Model file for the job. Use its own axes, mm. A direction names the side the tool comes from. Coordinates: 2 decimals unless noted, no trailing zeros. Write each loop counter-clockwise with the first axis right and the second up, starting at its lowest first coordinate (ties: lowest second). Pieces come first, ordered by that corner, then holes. Notation, with made-up numbers: M 37,84.5 L 81,84.5 A25 cw 81,98.5 Z; hole C 63.25,39 d5. An arc over 180 degrees is marked long. Answer in a Markdown table with one row per item. Add a question column.
```python
from build123d import *

# Parameters (mm, degrees)
ESBO_O2_W                = 173
ESBO_O2_H                = 45.2
RESSALTO_EXTRUS_O2_DEPTH = 65.2
ESBO_O3_R                = 57.970457698
RESSALTO_EXTRUS_O3_DEPTH = 20
RESSALTO_EXTRUS_O4_START = -45.2
RESSALTO_EXTRUS_O4_DEPTH = 45.2


# Read off the part's stored shape, not the designer's step: Ressalto-extrusão4
with BuildPart() as part:
    # Esboço2 → Ressalto-extrusão2 (new, symmetric)
    with BuildSketch(Plane(origin=(0, 0, 0), x_dir=(1, 0, 0), z_dir=(0, 1, 0))):
        Rectangle(ESBO_O2_W, ESBO_O2_H)
    extrude(amount=RESSALTO_EXTRUS_O2_DEPTH, both=True)

    # Esboço3 → Ressalto-extrusão3 (add)
    with BuildSketch(Plane.XY.offset(22.6)):
        with Locations((-17.919078136, -1.804884681)):
            Circle(ESBO_O3_R)
    extrude(amount=RESSALTO_EXTRUS_O3_DEPTH)

    # Ressalto-extrusão4 outline → Ressalto-extrusão4 (add)
    with BuildSketch(Plane.XY.offset(22.6).offset(RESSALTO_EXTRUS_O4_START)):
        with BuildLine():
            Line((102.68744208, 77.672367144), (93.883087158, 68.853831482))
            Line((93.883087158, 68.853831482), (92.930908203, 67.948153687))
            Line((92.930908203, 67.948153687), (92.052246094, 67.253565979))
            Line((92.052246094, 67.253565979), (91.246276855, 66.845568848))
            Line((91.246276855, 66.845568848), (90.411560059, 66.271777344))
            Line((90.411560059, 66.271777344), (87.657562256, 65.351000977))
            Line((87.657562256, 65.351000977), (86.5, 65.2))
            Line((86.5, 65.2), (86.5, -65.2))
            Line((86.5, -65.2), (93.839447021, -65.336684036))
            Line((93.839447021, -65.336684036), (95.128540039, -65.774876404))
            Line((95.128540039, -65.774876404), (95.626312256, -65.865172195))
            Line((95.626312256, -65.865172195), (97.838317871, -67.1335495))
            Line((97.838317871, -67.1335495), (103.111968994, -71.512766647))
            Line((103.111968994, -71.512766647), (104.284179687, -71.844658661))
            Line((104.284179687, -71.844658661), (105.016326904, -72.192253876))
            Line((105.016326904, -72.192253876), (106.758210561, -72.501532079))
            Line((106.758210561, -72.501532079), (127.042376704, -72.501532079))
            Line((127.042376704, -72.501532079), (128.748016357, -72.237250137))
            Line((128.748016357, -72.237250137), (129.333953857, -71.920157242))
            Line((129.333953857, -71.920157242), (130.505584717, -71.542965698))
            Line((130.505584717, -71.542965698), (132.116973877, -70.621580887))
            Line((132.116973877, -70.621580887), (132.908325195, -70.379986572))
            Line((132.908325195, -70.379986572), (133.581878662, -70.455786514))
            ThreePointArc((133.581878662, -70.455786514), (136.426489502, -71.540170383), (139.104858398, -70.09309082))
            Line((139.104858398, -70.09309082), (144.451446533, -57.847529221))
            ThreePointArc((144.451446533, -57.847529221), (143.532086949, -55.594745414), (141.463348389, -54.313895035))
            Line((141.463348389, -54.313895035), (141.155700684, -53.921302605))
            Line((141.155700684, -53.921302605), (141.155700684, -52.985422897))
            Line((141.155700684, -52.985422897), (141.8878479, -50.116176057))
            Line((141.8878479, -50.116176057), (142.04901123, -47.851521599))
            Line((142.04901123, -47.851521599), (142.561706543, -42.41532402))
            Line((142.561706543, -42.41532402), (142.217758179, -36.926730919))
            Line((142.217758179, -36.926730919), (141.770965576, -33.015906143))
            Line((141.770965576, -33.015906143), (131.194091797, 22.060099792))
            Line((131.194091797, 22.060099792), (130.901397705, 24.174060059))
            Line((130.901397705, 24.174060059), (130.286132812, 26.96738739))
            Line((130.286132812, 26.96738739), (130.286132812, 31.270747375))
            Line((130.286132812, 31.270747375), (131.20904541, 35.347880554))
            Line((131.20904541, 35.347880554), (133.098449707, 39.741893005))
            Line((133.098449707, 39.741893005), (133.699371338, 41.055262756))
            Line((133.699371338, 41.055262756), (133.97769165, 41.886050415))
            Line((133.97769165, 41.886050415), (134.49041748, 42.821932983))
            Line((134.49041748, 42.821932983), (135.134979248, 44.815394592))
            Line((135.134979248, 44.815394592), (135.427642822, 45.69118042))
            Line((135.427642822, 45.69118042), (135.632751465, 46.974353027))
            Line((135.632751465, 46.974353027), (135.60345459, 53.694026184))
            Line((135.60345459, 53.694026184), (135.515838623, 59.205119324))
            Line((135.515838623, 59.205119324), (135.354400635, 60.790583801))
            Line((135.354400635, 60.790583801), (134.665893555, 63.161540222))
            Line((134.665893555, 63.161540222), (134.54901123, 63.659831238))
            Line((134.54901123, 63.659831238), (134.065307617, 64.490313721))
            Line((134.065307617, 64.490313721), (133.684417725, 65.441600037))
            Line((133.684417725, 65.441600037), (132.36630249, 67.208262634))
            Line((132.36630249, 67.208262634), (131.38482666, 68.355540466))
            Line((131.38482666, 68.355540466), (123.254638672, 76.434184265))
            Line((123.254638672, 76.434184265), (122.302154541, 77.249568176))
            Line((122.302154541, 77.249568176), (120.544555664, 78.200854492))
            Line((120.544555664, 78.200854492), (120.134399414, 78.668643188))
            ThreePointArc((120.134399414, 78.668643188), (119.353688391, 81.369611441), (116.808776855, 82.5646698))
            Line((116.808776855, 82.5646698), (106.483274703, 82.583373499))
            ThreePointArc((106.483274703, 82.583373499), (103.379795658, 81.059678188), (102.68744208, 77.672367144))
        make_face()
        with BuildLine():
            Line((-128.748016357, -72.237250137), (-127.042376704, -72.501532079))
            Line((-127.042376704, -72.501532079), (-106.758210561, -72.501532079))
            Line((-106.758210561, -72.501532079), (-105.016326904, -72.192253876))
            Line((-105.016326904, -72.192253876), (-104.284179688, -71.844658661))
            Line((-104.284179688, -71.844658661), (-103.111968994, -71.512766647))
            Line((-103.111968994, -71.512766647), (-97.838317871, -67.1335495))
            Line((-97.838317871, -67.1335495), (-95.626312256, -65.865172195))
            Line((-95.626312256, -65.865172195), (-95.128540039, -65.774876404))
            Line((-95.128540039, -65.774876404), (-93.839447021, -65.336684036))
            Line((-93.839447021, -65.336684036), (-86.5, -65.2))
            Line((-86.5, -65.2), (-86.5, 65.2))
            Line((-86.5, 65.2), (-87.657562256, 65.351000977))
            Line((-87.657562256, 65.351000977), (-90.411560059, 66.271777344))
            Line((-90.411560059, 66.271777344), (-91.246276855, 66.845568848))
            Line((-91.246276855, 66.845568848), (-92.052246094, 67.253565979))
            Line((-92.052246094, 67.253565979), (-92.930908203, 67.948153687))
            Line((-92.930908203, 67.948153687), (-93.883087158, 68.853831482))
            Line((-93.883087158, 68.853831482), (-102.68744208, 77.672367144))
            ThreePointArc((-102.68744208, 77.672367144), (-103.379795658, 81.059678188), (-106.483274703, 82.583373499))
            Line((-106.483274703, 82.583373499), (-116.808776855, 82.5646698))
            ThreePointArc((-116.808776855, 82.5646698), (-119.353688391, 81.369611441), (-120.134399414, 78.668643188))
            Line((-120.134399414, 78.668643188), (-120.544555664, 78.200854492))
            Line((-120.544555664, 78.200854492), (-122.302154541, 77.249568176))
            Line((-122.302154541, 77.249568176), (-123.254638672, 76.434184265))
            Line((-123.254638672, 76.434184265), (-131.38482666, 68.355540466))
            Line((-131.38482666, 68.355540466), (-132.36630249, 67.208262634))
            Line((-132.36630249, 67.208262634), (-133.684417725, 65.441600037))
            Line((-133.684417725, 65.441600037), (-134.065307617, 64.490313721))
            Line((-134.065307617, 64.490313721), (-134.54901123, 63.659831238))
            Line((-134.54901123, 63.659831238), (-134.665893555, 63.161540222))
            Line((-134.665893555, 63.161540222), (-135.354400635, 60.790583801))
            Line((-135.354400635, 60.790583801), (-135.515838623, 59.205119324))
            Line((-135.515838623, 59.205119324), (-135.60345459, 53.694026184))
            Line((-135.60345459, 53.694026184), (-135.632751465, 46.974353027))
            Line((-135.632751465, 46.974353027), (-135.427642822, 45.69118042))
            Line((-135.427642822, 45.69118042), (-135.134979248, 44.815394592))
            Line((-135.134979248, 44.815394592), (-134.49041748, 42.821932983))
            Line((-134.49041748, 42.821932983), (-133.97769165, 41.886050415))
            Line((-133.97769165, 41.886050415), (-133.699371338, 41.055262756))
            Line((-133.699371338, 41.055262756), (-133.098449707, 39.741893005))
            Line((-133.098449707, 39.741893005), (-131.20904541, 35.347880554))
            Line((-131.20904541, 35.347880554), (-130.286132813, 31.270747375))
            Line((-130.286132813, 31.270747375), (-130.286132812, 26.96738739))
            Line((-130.286132812, 26.96738739), (-130.901397705, 24.174060059))
            Line((-130.901397705, 24.174060059), (-131.194091797, 22.060099792))
            Line((-131.194091797, 22.060099792), (-141.770965576, -33.015906143))
            Line((-141.770965576, -33.015906143), (-142.217758179, -36.926730919))
            Line((-142.217758179, -36.926730919), (-142.561706543, -42.41532402))
            Line((-142.561706543, -42.41532402), (-142.04901123, -47.851521599))
            Line((-142.04901123, -47.851521599), (-141.8878479, -50.116176057))
            Line((-141.8878479, -50.116176057), (-141.155700684, -52.985422897))
            Line((-141.155700684, -52.985422897), (-141.155700684, -53.921302605))
            Line((-141.155700684, -53.921302605), (-141.463348389, -54.313895035))
            ThreePointArc((-141.463348389, -54.313895035), (-143.532086949, -55.594745414), (-144.451446533, -57.847529221))
            Line((-144.451446533, -57.847529221), (-139.104858398, -70.09309082))
            ThreePointArc((-139.104858398, -70.09309082), (-136.426489502, -71.540170383), (-133.581878662, -70.455786514))
            Line((-133.581878662, -70.455786514), (-132.908325195, -70.379986572))
            Line((-132.908325195, -70.379986572), (-132.116973877, -70.621580887))
            Line((-132.116973877, -70.621580887), (-130.505584717, -71.542965698))
            Line((-130.505584717, -71.542965698), (-129.333953857, -71.920157242))
            Line((-129.333953857, -71.920157242), (-128.748016357, -72.237250137))
        make_face()
    extrude(amount=RESSALTO_EXTRUS_O4_DEPTH)


solid = part.part
```
1) Slice it at B-B (x = 36). Give the cut face in (y, z).
2) Slice it at C-C (z = 34.5). Give the cut face in (x, y), then the cut area to 3 significant figures.
3) Drill centre lines: probe 1 along Y at (x, z) = (-29, 8.5); probe 2 along Z at (x, y) = (100.5, 24.5); probe 3 along X at (y, z) = (-66, 20.5). Where is each one in solid material? Low to high.
4) Two-plate mould, pull along Y, no slides. Class faces 1 (the face through (-142.31, -45.1, -0.32)), 2 (the face through (136.383, -71.543, -0.316)), 3 (the face through (-2, 6, -22.6)): released by +Y, released by -Y, zero draft, split by the parting line, or undercut.
5) Which spindle directions (+Z, -Z, +X, -X, +Y, -Y) get a long thin tool onto all of the face, cutting with end or side? Do faces 4 (the face through (100.438, -69.293, -0.316)), 5 (the face through (-136.41, -5.09, -0.32)), 6 (the face through (-142.387, -39.633, -0.316)). Say none if no direction does.
6) Slice it at D-D (x = 112). Give the cut face in (y, z), then the cut area to 3 significant figures.
7) Slice it at A-A (y = -4.5). Give the cut face in (x, z).
8) Flat gauge pins, fed straight in: pin 1 Ø4 at (x, z) = (16.5, 25) entering from -Y; pin 2 Ø3.5 at (y, z) = (28.5, -1) entering from -X; pin 3 Ø12 at (y, z) = (-32.5, 8) entering from -X. Where does each tip first touch, or does it go through?
Ans:
| question | item | result |
|---|---|---|
| 1 | outline | M -65.2,-22.6 L 65.2,-22.6 L 65.2,22.6 L 19.49,22.6 L 19.49,42.6 L -23.1,42.6 L -23.1,22.6 L -65.2,22.6 Z |
| 2 | outline | C -17.92,-1.8 d115.94 |
| 2 | area | 10,600 mm2 |
| 3 | probe 1 | y = -65.2 to 65.2 |
| 3 | probe 2 | z = -22.6 to 22.6 |
| 3 | probe 3 | x = -140.89 to -95.86, 95.86 to 140.89 |
| 4 | face 1 | undercut |
| 4 | face 2 | released by -Y |
| 4 | face 3 | zero draft |
| 5 | face 4 | +Z, -Z, -Y |
| 5 | face 5 | +Z, -Z, -X |
| 5 | face 6 | +Z, -Z, -X, +Y |
| 6 | outline | M -72.5,-22.6 L 82.57,-22.6 L 82.57,22.6 L -72.5,22.6 Z |
| 6 | area | 7,010 mm2 |
| 7 | outline | M -136.29,-22.6 L 136.29,-22.6 L 136.29,22.6 L 39.99,22.6 L 39.99,42.6 L -75.83,42.6 L -75.83,22.6 L -136.29,22.6 Z |
| 8 | pin 1 | stops at y = -49.86 |
| 8 | pin 2 | stops at x = -130.33 |
| 8 | pin 3 | stops at x = -142.32 |
